Could you check a few things on this drawing? It's one solid part, dimensions in mm from its lowest x, y, z. A direction names the side the tool comes from. Coordinates: 2 decimals unless noted, no trailing zeros. Order: outer loops, then holes, each group sorted by start corner. A loop starts at its lowest first (then second) coordinate and runs counter-clockwise, first axis right, second up. Notation, with made-up numbers: (-16, 25) -> (-8, 25) arc R12 ccw to (-8, 31) -> close; hole circle Ø10 at (-27.75, 46.25). An arc over 180 degrees is marked (long way). Use a Markdown table: item, result. Add a question column.
1. For pin 1 Ø1.5 at (x, y) = (16.5, 2) entering from -Z; pin 2 Ø0.9 at (y, z) = (1, 1) entering from +X; pin 3 Ø0.9 at (x, y) = (15, 1.5) entering from +Z; pin 4 Ø1.5 at (y, z) = (2, 1.5) entering from -X, each with a flat end and sliding along its axis, tell me the tip position at first contact or that it passes through.
2. For the marked faces 4, 5 and 6, which set-ups out of +Z, -Z, +X, -X, +Y, -Y let a thin tool reach every point of the face, with its end or its side?
3. Suppose I cut it at A-A, the plane y = 2. List the corners of the cut face in (x, z) for me, then the cut area to 3 significant figures.
4. We'd pull the mould along Z, two halves only. Please class the marked faces 1, 2 and 3: pulls with the +Z half, pulls with the -Z half, needs draft (parallel to the pull), parting line crosses it, or undercut.
5. Suppose I cut it at B-B, the plane z = 5.75. List the corners of the cut face in (x, y) for me.
6. Suppose I cut it at C-C, the plane z = 10.25. List the corners of the cut face in (x, y) for me, then the cut area to 3 significant figures.
7. If I drill on line 1 along X through (y, z) = (2.35, 2.75); line 2 along Z through (x, y) = (17.5, 0.4); line 3 along X through (y, z) = (2.2, 5.25), over which ranges is the centre line in solid material (lowest first)? Write a range as from..to.
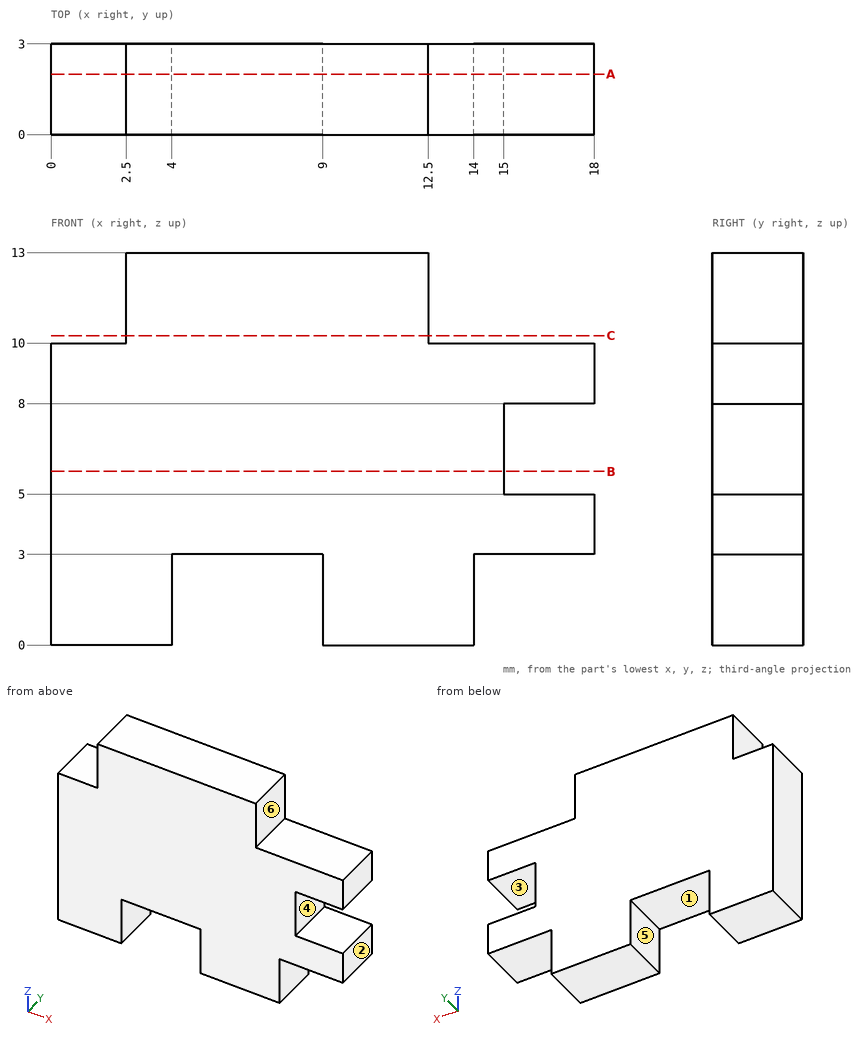
Worked out:
| question | item | result |
|---|---|---|
| 1 | pin 1 | stops at z = 3 |
| 1 | pin 2 | stops at x = 14 |
| 1 | pin 3 | stops at z = 10 |
| 1 | pin 4 | stops at x = 0 |
| 2 | face 4 | +X, +Y, -Y |
| 2 | face 5 | -Z, +Y, -Y |
| 2 | face 6 | +Z, +X, +Y, -Y |
| 3 | outline | (0, 0) -> (4, 0) -> (4, 3) -> (9, 3) -> (9, 0) -> (14, 0) -> (14, 3) -> (18, 3) -> (18, 5) -> (15, 5) -> (15, 8) -> (18, 8) -> (18, 10) -> (12.5, 10) -> (12.5, 13) -> (2.5, 13) -> (2.5, 10) -> (0, 10) -> close |
| 3 | area | 174 mm² |
| 4 | face 1 | pulls with the -Z half |
| 4 | face 2 | needs draft |
| 4 | face 3 | undercut |
| 5 | outline | (0, 0) -> (15, 0) -> (15, 3) -> (0, 3) -> close |
| 6 | outline | (2.5, 0) -> (12.5, 0) -> (12.5, 3) -> (2.5, 3) -> close |
| 6 | area | 30.0 mm² |
| 7 | line 1 | x = 0..4, 9..14 |
| 7 | line 2 | z = 3..5, 8..10 |
| 7 | line 3 | x = 0..15 |
